from build123d import *

# Parameters (mm, degrees)
SKETCH1_R               = 5
SKETCH1_R_2             = 4
BOSS_EXTRUDE1_DEPTH     = 60
SKETCH1_4_R             = 5
SKETCH1_4_R_2           = 4
CUT_EXTRUDE1_DEPTH      = 10
CUT_EXTRUDE2_START      = 40
SKETCH1_5_R             = 4
CUT_EXTRUDE2_DEPTH      = 20
CUT_EXTRUDE3_DEPTH      = 61.415229868
CUT_EXTRUDE3_DEPTH_BACK = 61.415229868


with BuildPart() as part:
    # Sketch1 → Boss-Extrude1 (new body)
    # profile 1 of 2: a face of its own
    with BuildSketch(Plane.XY):
        Circle(SKETCH1_R)
        Circle(SKETCH1_R_2, mode=Mode.SUBTRACT)
    # profile 2 of 2: a face of its own
    with BuildSketch(Plane.XY):
        Circle(SKETCH1_R_2)
    extrude(amount=BOSS_EXTRUDE1_DEPTH)

    # Sketch1_4 → Cut-Extrude1 (cut)
    with BuildSketch(Plane.XY):
        Circle(SKETCH1_4_R)
        Circle(SKETCH1_4_R_2, mode=Mode.SUBTRACT)
    extrude(amount=CUT_EXTRUDE1_DEPTH, mode=Mode.SUBTRACT)

    # Sketch1_5 → Cut-Extrude2 (cut)
    with BuildSketch(Plane.XY.offset(CUT_EXTRUDE2_START)):
        Circle(SKETCH1_5_R)
    extrude(amount=CUT_EXTRUDE2_DEPTH, mode=Mode.SUBTRACT)

    # Sketch2 → Cut-Extrude3 (cut, two sides: drawn at the far end of the back side and taken through both)
    with BuildSketch(Plane(origin=(0, 0, 0), x_dir=(1, 0, 0), z_dir=(0, 1, 0)).offset(-CUT_EXTRUDE3_DEPTH_BACK)):
        with BuildLine():
            Line((2, -48), (2, -55))
            ThreePointArc((2, -55), (0, -57), (-2, -55))
            Line((-2, -55), (-2, -48))
            ThreePointArc((-2, -48), (0, -46), (2, -48))
        make_face()
    extrude(amount=CUT_EXTRUDE3_DEPTH + CUT_EXTRUDE3_DEPTH_BACK, mode=Mode.SUBTRACT)


solid = part.part
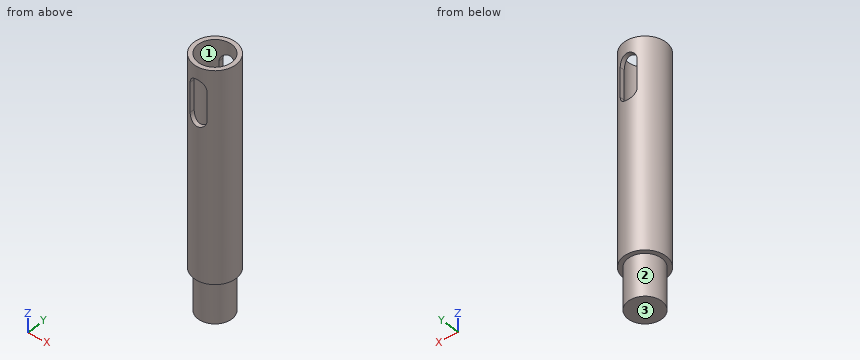
Check sheet for the modelled part. Datum: model origin and axes. Units: mm. Face numbers are marked on the shaded views. Give positions to 0.01 mm unless a question says otherwise; leave off trailing zeros. Loops run counter-clockwise (first coordinate to the right, second up) from the corner with the lowest first, then second, coordinate; pieces in that order, holes last. Notation, with made-up numbers: M 64.5,-19.5 L 108.5,-19.5 A17 cw 108.5,-15.5 Z; hole C 74.5,65 d11. An arc over 180 degrees is marked long. Return JSON: item names as keys, results as strings. Group by question number.
1. Cross-section at D-D on x = -3.5. Record the boundary of the cut face in (y, z).
2. Cross-section at A-A on x = 1. Record the boundary of the cut face in (y, z), plus the area to 3 significant figures.
3. Go/stop test with flat-tipped pins: pin 1 (4 mm diameter, centred on x = 1.5, y = -1, fed in from +Z); pin 2 (4 mm diameter, centred on y = -3, z = 13.5, fed in from -X); pin 3 (0.9 mm diameter, centred on y = 4, z = 51.5, fed in from -X). Record where each tip stops, or that it passes through.
4. Cross-section at B-B on y = 0. Record the boundary of the cut face in (x, z), plus the area to 3 significant figures.
5. Cross-section at C-C on z = 43.5. Record the boundary of the cut face in (x, y), plus the area to 3 significant figures.
6. Mould release check, pull along Y, two halves, no side actions. Record for the marked faces 1, 2 and 3: released by +Y, released by -Y, zero draft, split by the parting line, or undercut.
7. Thickness scan on L1, parallel to Y at x = 0, z = 45.25; L2, parallel to Y at x = 1.5, z = 43; L3, parallel to Z at x = 0.25, y = -2. Record the ranges inside material, lowest first.
Return value:
{
 "1": {"outline": "M -3.57,10 L -1.94,10 L -1.94,0 L 1.94,0 L 1.94,10 L 3.57,10 L 3.57,60 L 1.94,60 L 1.94,40 L -1.94,40 L -1.94,60 L -3.57,60 Z"},
 "2": {"outline": "M -4.9,10 L -3.87,10 L -3.87,0 L 3.87,0 L 3.87,10 L 4.9,10 L 4.9,46.27 L 3.87,46.27 L 3.87,40 L -3.87,40 L -3.87,46.27 L -4.9,46.27 Z; M -4.9,56.73 L -3.87,56.73 L -3.87,60 L -4.9,60 Z; M 3.87,56.73 L 4.9,56.73 L 4.9,60 L 3.87,60 Z", "area": "391 mm^2"},
 "3": {"pin 1": "z = 40", "pin 2": "x = -4.9", "pin 3": "x = -3.52"},
 "4": {"outline": "M -5,10 L -4,10 L -4,0 L 4,0 L 4,10 L 5,10 L 5,60 L 4,60 L 4,40 L -4,40 L -4,60 L -5,60 Z", "area": "420 mm^2"},
 "5": {"outline": "C 0,0 d10; hole C 0,0 d8", "area": "28.3 mm^2"},
 "6": {"face 1": "undercut", "face 2": "split by the parting line", "face 3": "zero draft"},
 "7": {"L1": "-5 to -4, 4 to 5", "L2": "-4.77 to -3.71, 3.71 to 4.77", "L3": "0 to 40"}
}
